from build123d import *

# Parameters (mm, degrees)
F0_W     = 360
F0_H     = 100
F1_DEPTH = 15
F3_DEPTH = 15


with BuildPart() as f1:
    # F0 (on Front) → F1 (new body)
    with BuildSketch(Plane.XZ):
        with Locations((-12.363208, -2.984696)):
            Rectangle(F0_W, F0_H)
    extrude(amount=F1_DEPTH)

    # F2 (on face) → F3 (intersect, through all)
    with BuildSketch(Plane.XZ.offset(15)):
        Polygon((-182.363208, 47.015304), (-192.363208, 47.015304), (-192.363208, -52.984696), (167.636792, -52.984696), (167.636792, 47.015304), (157.636792, 47.015304), (155.136792, -32.984696), (135.136792, -32.984696), (132.636792, 47.015304), (122.636792, 47.015304), (120.136792, -32.984696), (100.136792, -32.984696), (97.636792, 47.015304), (87.636792, 47.015304), (85.136792, -32.984696), (65.136792, -32.984696), (62.636792, 47.015304), (52.636792, 47.015304), (50.136792, -32.984696), (30.136792, -32.984696), (27.636792, 47.015304), (17.636792, 47.015304), (15.136792, -32.984696), (-4.863208, -32.984696), (-7.363208, 47.015304), (-17.363208, 47.015304), (-19.863208, -32.984696), (-39.863208, -32.984696), (-42.363208, 47.015304), (-52.363208, 47.015304), (-54.863208, -32.984696), (-74.863208, -32.984696), (-77.363208, 47.015304), (-87.363208, 47.015304), (-89.863208, -32.984696), (-109.863208, -32.984696), (-112.363208, 47.015304), (-122.363208, 47.015304), (-124.863208, -32.984696), (-144.863208, -32.984696), (-147.363208, 47.015304), (-157.363208, 47.015304), (-159.863208, -32.984696), (-179.863208, -32.984696), align=None)
    extrude(amount=-F3_DEPTH, mode=Mode.INTERSECT)


solid = f1.part
The listing builds one solid part. Answer for the finished solid, in the listing's coordinates (mm). A direction names the side the tool comes from. Round coordinates to 2 decimals unless told otherwise and drop trailing zeros. Write each loop counter-clockwise with the first axis right and the second up, starting at its lowest first coordinate (ties: lowest second). Pieces come first, ordered by that corner, then holes. Notation, with made-up numbers: M 35.25,45.25 L 39.25,45.25 A10 cw 39.25,53.25 Z; hole C 79.25,7.5 d7. An arc over 180 degrees is marked long. Write each question's results on one line, items separated by ' | '. Start each with the question number.
(1) The part is cut by section B-B, the plane x = -61.5. Write down the section's boundary in (y, z), and give its area (3 significant figures).
(2) Determine the mould class of faces 3 (the flat face through (-30, -8, -32.985)), 4 (the flat face through (-187, -7, 47.015)) for opening direction X: +X half, -X half, draft (parallel to the pull), parting line (faces both ways), or undercut.
(3) This flat-tipped pin is pushed along its axis until it touches: P1, Ø4.5, axis at x = 3.5, y = -6.5, coming from the +Z side. Where does it stop, or does it pass through?
(4) Find the intervals of material crossed by line 1 (Z direction, x = -33.5, y = -7.5), in increasing order.
(5) The part is cut by section A-A, the plane z = 9. Give the number of separate pieces and of enclosed holes in the cut face, and give its area (3 significant figures).
(6) For faces 1 (the flat face through (-65, -8, -32.985)), 2 (the flat face through (23, -8, 47.015)), determine the directions among +Z, -Z, +X, -X, +Y, -Y from which every point of the face is accessible in a straight line to the end or side of a thin tool.
Worked answers:
1) outline: M -15,-52.98 L 0,-52.98 L 0,-32.98 L -15,-32.98 Z | area: 300 mm²
2) face 3: undercut | face 4: draft
3) P1: stops at z = -32.98
4) line 1: z = -52.98 to -32.98
5) separate pieces: 11 | enclosed holes: 0 | area: 2,010 mm²
6) face 1: +Z, +Y, -Y | face 2: +Z, +X, -X, +Y, -Y
